Check sheet for the drawn part. Datum: minimum x, y, z corner. Units: mm. Round coordinates to 2 decimals unless told otherwise and drop trailing zeros. Write each loop counter-clockwise with the first axis right and the second up, starting at its lowest first coordinate (ties: lowest second). Pieces come first, ordered by that corner, then holes. Notation, with made-up numbers: (69.5, -22) - (100.5, -22) arc R33 ccw to (100.5, 12) - close; hole circle Ø2 at (26.25, 45.25). An arc over 180 degrees is marked (long way). Answer as a JSON object with one key per item and string values. Group by question number.
Item 1: Gauge pin test, flat end, axial feed: P1, Ø1, axis at y = 88.5, z = 24.5, coming from the -X side. Record the tip position at first contact, or that the pin passes through.
Item 2: Sectioned sample at A-A on x = 37.99. Record the boundary of the cut face in (y, z) (1 decimal), plus the area to 3 significant figures.
Item 3: Release check for a two-part mould opening along X. For the marked faces 1, 2, 3 and 4 record: pulls with the +X half, pulls with the -X half, needs draft (parallel to the pull), parting line crosses it, or undercut.
Item 4: Sectioned sample at B-B on z = 25. Record the boundary of the cut face in (x, y) (1 decimal).
Item 5: Thickness scan on line 1 (Z direction, x = 37.99, y = 59) (1 decimal); line 2 (X direction, y = 49.5, z = 29) (1 decimal); line 3 (Z direction, x = 21, y = 17) (1 decimal). Record the ranges inside material, lowest first.
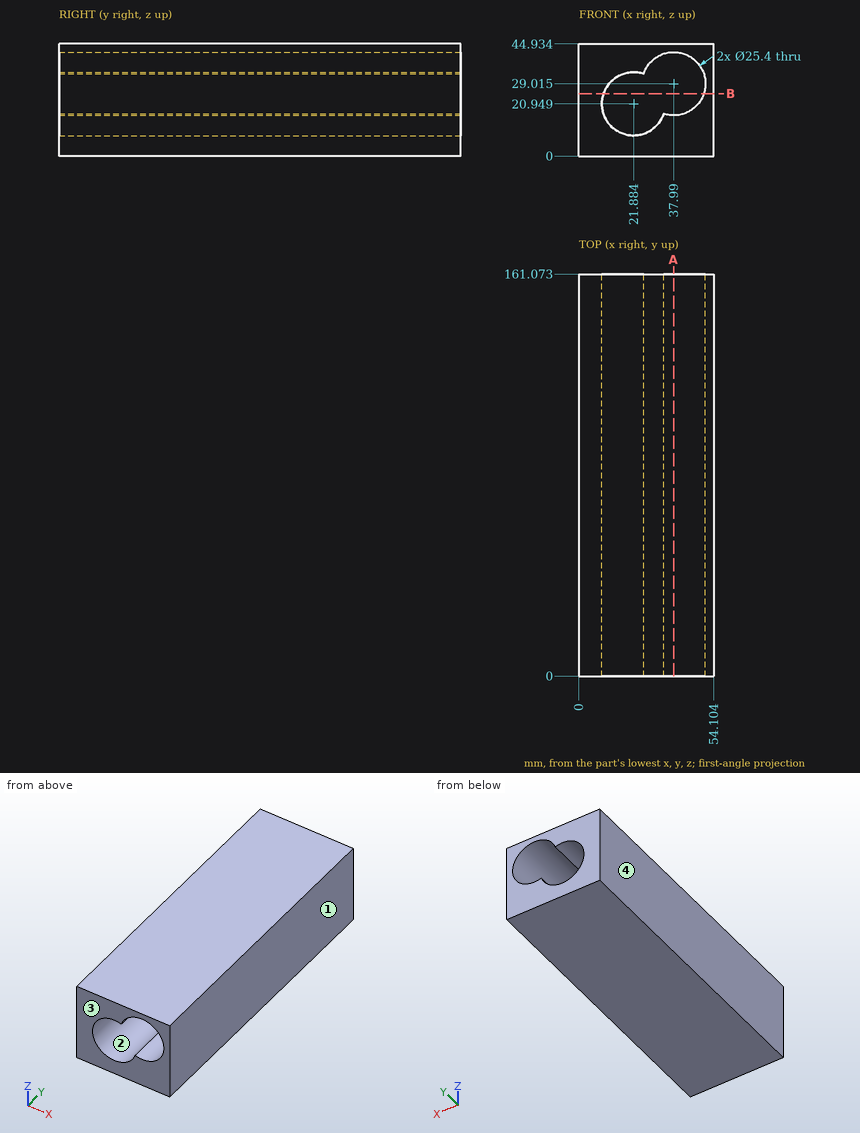
Completed:
{
 "1": {"P1": "x = 0"},
 "2": {"outline": "(0, 0) - (161.1, 0) - (161.1, 16.3) - (0, 16.3) - close; (0, 41.7) - (161.1, 41.7) - (161.1, 44.9) - (0, 44.9) - close", "area": "3,150 mm²"},
 "3": {"face 1": "pulls with the +X half", "face 2": "undercut", "face 3": "needs draft", "face 4": "pulls with the -X half"},
 "4": {"outline": "(0, 0) - (9.8, 0) - (9.8, 161.1) - (0, 161.1) - close; (50, 0) - (54.1, 0) - (54.1, 161.1) - (50, 161.1) - close"},
 "5": {"line 1": "0 to 16.3, 41.7 to 44.9", "line 2": "0 to 12.1, 50.7 to 54.1", "line 3": "0 to 8.3, 33.6 to 44.9"}
}
